Model file for the job. Use its own axes, mm. Face numbers are marked on the shaded views. A direction names the side the tool comes from. Round coordinates to 2 decimals unless told otherwise and drop trailing zeros. Loops run counter-clockwise (first coordinate to the right, second up) from the corner with the lowest first, then second, coordinate; pieces in that order, holes last. Notation, with made-up numbers: M 28,-30.5 L 83,-30.5 A30 cw 83,-4.5 Z; hole C -19.75,12.5 d9. An arc over 180 degrees is marked long. Use a Markdown table: item, result. Add a question column.
Q1. Cut at A-A (z = 8.25). Give the cut face in (x, y), plus the area to 3 significant figures.
Q2. Probe line 1 (X direction, y = 1, z = 6.5); line 2 (Y direction, x = 11, z = -3.25); line 3 (Z direction, x = 3.5, y = 1). List the from-to ranges inside material, lowest first. Write a range as from..to.
Q3. Cut at B-B (z = -1). Give the cut face in (x, y).
Q4. Cut at C-C (y = 3.5). Give the cut face in (x, z), plus the area to 3 significant figures.
Q5. Mould opens along Z. For the marked faces 4, 5 and 6 say: +Z half, -Z half, draft (parallel to the pull), parting line (faces both ways), or undercut.
Q6. Pin check, flat tips, straight feed: pin 1 (6 mm diameter, centred on x = 5.5, z = -7, fed in from -Y); pin 2 (9 mm diameter, centred on x = -4.5, z = -0.5, fed in from +Y); pin 3 (6 mm diameter, centred on y = -2, z = 3.5, fed in from -X); pin 4 (1.6 mm diameter, centred on x = -2, y = 1.5, fed in from -Z). Stop position of each tip, or through.
Q7. Cut at D-D (x = -4.75). Give the cut face in (y, z), plus the area to 3 significant figures.
Q8. Tool access for the marked faces 1, 2 and 3: list every direction of +Z, -Z, +X, -X, +Y, -Y with a clear straight run to the whole face (end or side of a thin tool).
Autodesk Inventor part; units mm, degrees
ref_plane "YZ Plane" through (0, 0, 0) normal (1, 0, 0) x (0, 1, 0)
ref_plane "XZ Plane" through (0, 0, 0) normal (0, 1, 0) x (-1, 0, 0)
ref_plane "XY Plane" through (0, 0, 0) normal (0, 0, 1) x (1, 0, 0)
sketch "Sketch1" plane through (0, 0, 0) normal (0, 1, 0) x (-1, 0, 0)
  line L0 (12.5, 9.25) -> (-12.5, 9.25)
  line L1 (-12.5, 9.25) -> (-12.5, -9.25)
  line L2 (-12.5, -9.25) -> (12.5, -9.25)
  line L3 (12.5, -9.25) -> (12.5, 9.25)
  line L4 (12.5, 9.25) -> (-12.5, -9.25) construction
  line L5 (-12.5, 9.25) -> (12.5, -9.25) construction
  line L6 (8, -4) -> (-8, -4)
  line L7 (-8, 4) -> (8, 4)
  line L8 (-17.5, 0) -> (17.5, 0)
  line L9 (8, -4) -> (8, -9.25)
  line L10 (8, 4) -> (8, 9.25)
  line L11 (-8, -4) -> (-8, -9.25)
  line L12 (-8, 4) -> (-8, 9.25)
  line L13 (0, -12.95) -> (0, 12.95)
  point P0 (0, 0)
  dimension "d0" = 25
  dimension "d1" = 18.5
  dimension "d24" = 8
  dimension "d25" = 16
extrude "Extrusion1" add sketch "Sketch1" along normal blind 2 contours L3 L8 L13 L7 L10 L0 | L3 L2 L9 L6 L13 L8 | L13 L6 L11 L2 L1 L8 | L8 L1 L0 L12 L7 L13
sketch "Sketch2" plane through (0, 2, 0) normal (0, 1, 0) x (1, 0, 0)
  line L0 (17.5, 0) -> (-17.5, 0)
  line L1 (0, 12.95) -> (0, -12.95)
  line L2 (-10, -6.25) -> (10, -6.25) construction
  line L3 (10, -6.25) -> (10, 6.25) construction
  line L4 (10, 6.25) -> (-10, 6.25) construction
  line L5 (-10, 6.25) -> (-10, -6.25) construction
  line L6 (-10, -6.25) -> (10, 6.25) construction
  line L7 (10, -6.25) -> (-10, 6.25) construction
  line L8 (-10, 0) -> (10, 0) construction
  circle A0 centre (10, -6.25) radius 1.05
  circle A1 centre (10, 6.25) radius 1.05
  circle A2 centre (-10, 6.25) radius 1.05
  circle A3 centre (-10, -6.25) radius 1.05
  point P0 (0, 0)
  dimension "d5" = 20
  dimension "d6" = 12.5
  dimension "d10" = 2.1
extrude "Extrusion2" add sketch "Sketch2" along normal blind 5
sketch "Sketch5" plane through (0, 0, 0) normal (0, -1, 0) x (1, 0, 0)
  line L0 (0, 12.95) -> (0, -12.95)
  line L1 (-17.5, 0) -> (17.5, 0)
  circle A0 centre (-4.75, -1) radius 1.5
  circle A1 centre (4.75, -1) radius 1.5
  point P0 (0, 0)
  dimension "d26" = 3
  dimension "d27" = 3
  dimension "d28" = 1
  dimension "d29" = 9.5
extrude "Extrusion4" add sketch "Sketch5" along normal blind 5
fillet "Fillet1" radius 2 4 edges at (-8, 1, 4) (8, 1, 4) (8, 1, -4) (-8, 1, -4)
properties part number "IMU mount"
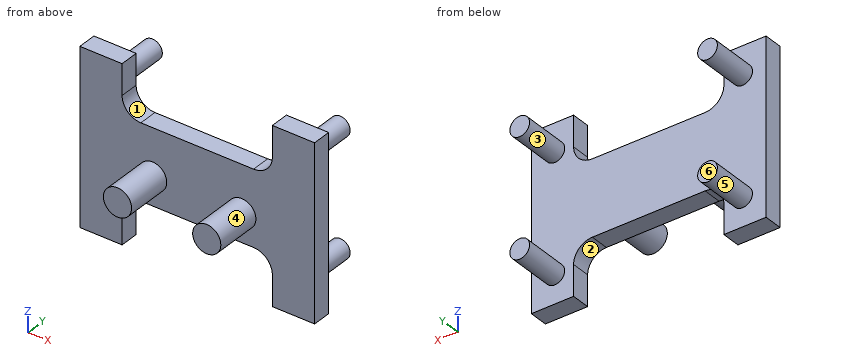
Checked values:
| question | item | result |
|---|---|---|
| 1 | outline | M -12.5,0 L -8,0 L -8,2 L -12.5,2 Z; M 8,0 L 12.5,0 L 12.5,2 L 8,2 Z |
| 1 | area | 18.0 mm^2 |
| 2 | line 1 | x = -12.5..-8, 8..12.5 |
| 2 | line 2 | y = 0..2 |
| 2 | line 3 | z = -4..4 |
| 3 | outline | M -12.5,0 L -6.25,0 L -6.25,-5 L -3.25,-5 L -3.25,0 L 3.25,0 L 3.25,-5 L 6.25,-5 L 6.25,0 L 12.5,0 L 12.5,2 L -12.5,2 Z |
| 4 | outline | C -10,-6.25 d2.1; C -10,6.25 d2.1; C 10,-6.25 d2.1; C 10,6.25 d2.1 |
| 4 | area | 13.9 mm^2 |
| 5 | face 4 | parting line |
| 5 | face 5 | undercut |
| 5 | face 6 | draft |
| 6 | pin 1 | stops at y = 0 |
| 6 | pin 2 | stops at y = 2 |
| 6 | pin 3 | stops at x = -12.5 |
| 6 | pin 4 | stops at z = -4 |
| 7 | outline | M -5,-2.5 L 0,-2.5 L 0,-4 L 2,-4 L 2,4 L 0,4 L 0,0.5 L -5,0.5 Z |
| 7 | area | 31.0 mm^2 |
| 8 | face 1 | +Z, +Y, -Y |
| 8 | face 2 | -Z, +Y, -Y |
| 8 | face 3 | +Y |
